The drawing under review shows one solid part. Ordinate dimensions are in mm from its lowest x, y, z. A direction names the side the tool comes from. Round coordinates to 2 decimals unless told otherwise and drop trailing zeros. Write each loop counter-clockwise with the first axis right and the second up, starting at its lowest first coordinate (ties: lowest second). Pieces come first, ordered by that corner, then holes. Notation, with made-up numbers: (-31, -9) -> (1, -9) arc R24 ccw to (1, 10) -> close; hole circle Ø8 at (58.25, -25.5). An arc over 180 degrees is marked (long way). Answer in a Markdown table with one row per item. Add a question column.
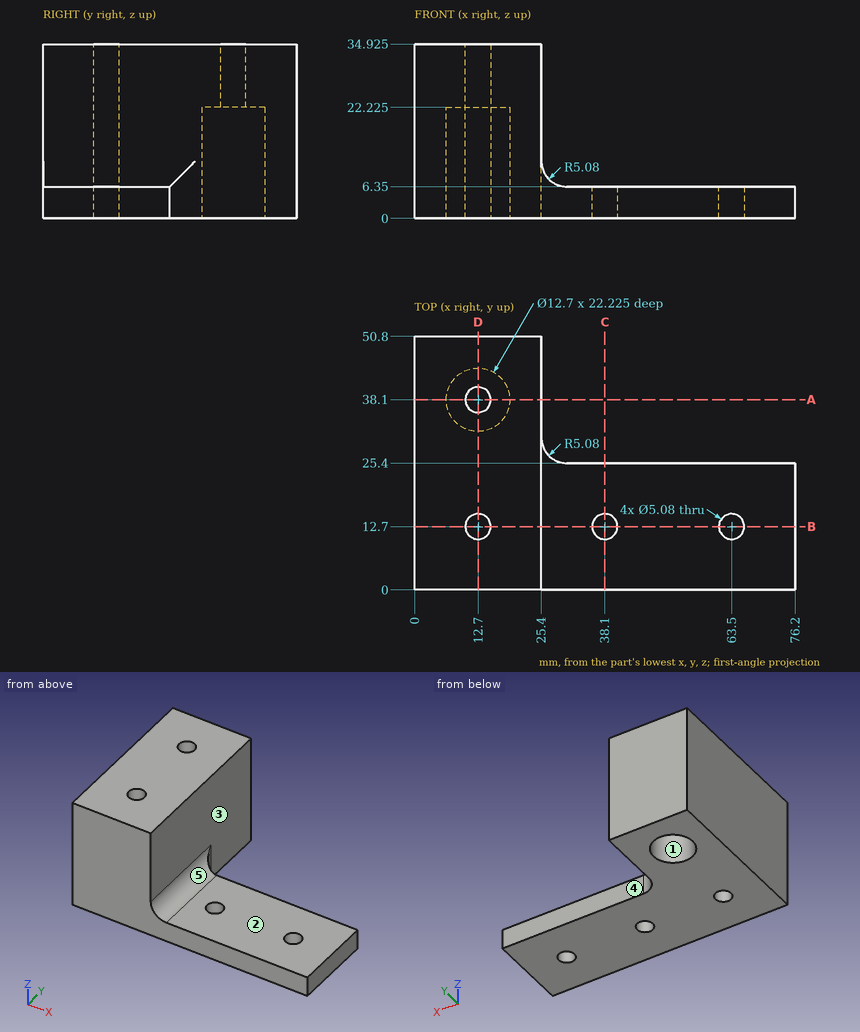
1. Add section C-C on x = 38.1. Write out the cut boundary in (y, z).
2. Add section D-D on x = 12.7. Write out the cut boundary in (y, z) (3 decimals), plus the area to 3 significant figures.
3. Insertion check: pin 1 Ø8 at (x, y) = (63.5, 12.7) entering from -Z; pin 2 Ø8 at (y, z) = (25.5, 28.5) entering from +X; pin 3 Ø6 at (x, y) = (48.5, 11) entering from +Z; pin 4 Ø4 at (x, y) = (10.5, 40.5) entering from -Z (3 decimals). Each pin has a flat end and moves straight along its axis. Give the tip position at first contact, or say it passes through.
4. Tool access review of the marked faces 4 and 5: name each direction out of +Z, -Z, +X, -X, +Y, -Y from which nothing blocks a thin tool from reaching the whole face with its end or side.
5. Add section B-B on y = 12.7. Write out the cut boundary in (x, z) (3 decimals).
6. For L1, parallel to Y at x = 12.7, z = 31; L2, parallel to Y at x = 63.5, z = 2.5; L3, parallel to Y at x = 12.7, z = 12, list the stretches that pass through material, from the lowest coordinate up.
7. Mouldability with a two-part tool opening along X and no side actions: class the marked faces 1, 2 and 3 as pulls with the +X half, pulls with the -X half, needs draft (parallel to the pull), parting line crosses it, or undercut.
8. Add section A-A on y = 38.1. Write out the cut boundary in (x, z) (3 decimals).
Filled in:
| question | item | result |
|---|---|---|
| 1 | outline | (0, 0) -> (10.16, 0) -> (10.16, 6.35) -> (0, 6.35) -> close; (15.24, 0) -> (25.4, 0) -> (25.4, 6.35) -> (15.24, 6.35) -> close |
| 2 | outline | (0, 0) -> (10.16, 0) -> (10.16, 34.925) -> (0, 34.925) -> close; (15.24, 0) -> (31.75, 0) -> (31.75, 22.225) -> (35.56, 22.225) -> (35.56, 34.925) -> (15.24, 34.925) -> close; (40.64, 22.225) -> (44.45, 22.225) -> (44.45, 0) -> (50.8, 0) -> (50.8, 34.925) -> (40.64, 34.925) -> close |
| 2 | area | 1,250 mm² |
| 3 | pin 1 | z = 0 |
| 3 | pin 2 | x = 25.4 |
| 3 | pin 3 | z = 6.35 |
| 3 | pin 4 | z = 22.225 |
| 4 | face 4 | +Z, -Z, +X, +Y |
| 4 | face 5 | +Z, +X, +Y, -Y |
| 5 | outline | (0, 0) -> (10.16, 0) -> (10.16, 34.925) -> (0, 34.925) -> close; (15.24, 0) -> (35.56, 0) -> (35.56, 6.35) -> (30.48, 6.35) arc R5.08 cw to (25.4, 11.43) -> (25.4, 34.925) -> (15.24, 34.925) -> close; (40.64, 0) -> (60.96, 0) -> (60.96, 6.35) -> (40.64, 6.35) -> close; (66.04, 0) -> (76.2, 0) -> (76.2, 6.35) -> (66.04, 6.35) -> close |
| 6 | L1 | 0 to 10.16, 15.24 to 35.56, 40.64 to 50.8 |
| 6 | L2 | 0 to 10.16, 15.24 to 25.4 |
| 6 | L3 | 0 to 10.16, 15.24 to 31.75, 44.45 to 50.8 |
| 7 | face 1 | undercut |
| 7 | face 2 | needs draft |
| 7 | face 3 | pulls with the +X half |
| 8 | outline | (0, 0) -> (6.35, 0) -> (6.35, 22.225) -> (10.16, 22.225) -> (10.16, 34.925) -> (0, 34.925) -> close; (15.24, 22.225) -> (19.05, 22.225) -> (19.05, 0) -> (25.4, 0) -> (25.4, 34.925) -> (15.24, 34.925) -> close |
